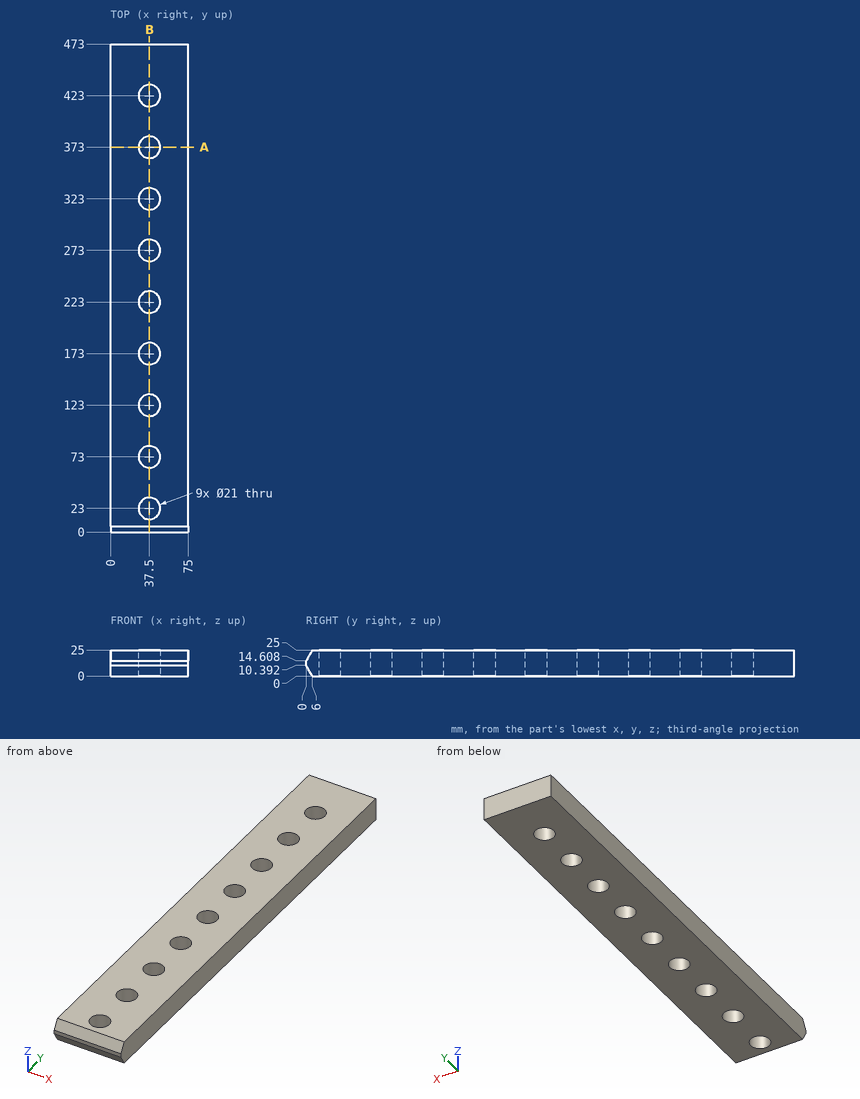
Check sheet for the drawn part. Datum: minimum x, y, z corner. Units: mm. Give positions to 0.01 mm unless a question says otherwise; leave off trailing zeros. Order: outer loops, then holes, each group sorted by start corner. A loop starts at its lowest first (then second) coordinate and runs counter-clockwise, first axis right, second up. Notation, with made-up numbers: (89, -2) -> (133, -2) arc R8 cw to (133, 9) -> close; hole circle Ø10 at (83, 75.5). An arc over 180 degrees is marked (long way). Return JSON: item names as keys, results as strings.
1. Cross-section at A-A, the plane y = 373. Record the cut outline in (x, z).
From the geometry:
{"outline": "(0, 0) -> (27, 0) -> (27, 25) -> (0, 25) -> close; (48, 0) -> (75, 0) -> (75, 25) -> (48, 25) -> close"}
2. Material ranges on probe 1 along X at (y, z) = (364, 11); probe 2 along X at (y, z) = (280.5, 16.25); probe 3 along Y at (x, z) = (50.5, 19) (1 decimal), recorded low to high. Write a range as [from, to].
From the geometry:
{"probe 1": "[0, 32.09], [42.91, 75]", "probe 2": "[0, 30.15], [44.85, 75]", "probe 3": "[2.5, 473]"}
3. Go/stop test with flat-tipped pins: P1, Ø5, axis at x = 35, z = 21, coming from the -Y side; P2, Ø19, axis at x = 37.5, y = 73, coming from the +Z side; P3, Ø3, axis at x = 52.5, z = 7, coming from the -Y side. Record where each tip stops, or that it passes through.
From the geometry:
{"P1": "y = 2.25", "P2": "through", "P3": "y = 1.09"}
4. Cross-section at B-B, the plane x = 37.5. Count the separate pieces of the cut face and the enclosed holes in it, plus the area to 3 significant figures.
From the geometry:
{"separate pieces": "10", "enclosed holes": "0", "area": "7,040 mm^2"}
